```python
from build123d import *

# Parameters (mm, degrees)
BOSS_EXTRUDE1_DEPTH = 20
BOSS_EXTRUDE2_DEPTH = 20
BOSS_EXTRUDE3_DEPTH = 20
SKETCH4_W           = 101.78899744
SKETCH4_H           = 2
SKETCH4_W_2         = 100
SKETCH4_W_3         = 60
SKETCH4_W_4         = 30.536699232
BOSS_EXTRUDE4_DEPTH = 10


with BuildPart() as part:
    # Sketch1 → Boss-Extrude1 (new body)
    with BuildSketch(Plane.XY):
        Polygon((0, 0), (0, 54), (100, 35), (100, 0), align=None)
    extrude(amount=BOSS_EXTRUDE1_DEPTH)

    # Sketch2 → Boss-Extrude2 (add)
    with BuildSketch(Plane.XY.offset(20)):
        Polygon((0, 54), (0, 0), (60, 0), (60, 42.6), align=None)
    extrude(amount=BOSS_EXTRUDE2_DEPTH)

    # Sketch3 → Boss-Extrude3 (add)
    with BuildSketch(Plane.XY.offset(40)):
        Polygon((0, 54), (0, 0), (30, 0), (30, 48.3), align=None)
    extrude(amount=BOSS_EXTRUDE3_DEPTH)

    # Sketch4 → Boss-Extrude4 (add)
    with BuildSketch(Plane(origin=(9.902519062, 52.118521378, 0), x_dir=(0.982424451701422, -0.1866606458232701, 0), z_dir=(0.1866606458232701, 0.982424451701422, 0))):
        with Locations((40.814823846, -1)):
            Rectangle(SKETCH4_W, SKETCH4_H)
        with Locations((39.920325126, -19)):
            Rectangle(SKETCH4_W_2, SKETCH4_H)
        with Locations((19.920325126, -39)):
            Rectangle(SKETCH4_W_3, SKETCH4_H)
        with Locations((5.188674742, -59)):
            Rectangle(SKETCH4_W_4, SKETCH4_H)
    extrude(amount=BOSS_EXTRUDE4_DEPTH)


solid = part.part
```
Build history of the part. All positions in model axes, mm. A direction names the side the tool comes from. Give positions to 0.01 mm unless a question says otherwise; leave off trailing zeros. Loops run counter-clockwise (first coordinate to the right, second up) from the corner with the lowest first, then second, coordinate; pieces in that order, holes last. Notation, with made-up numbers: (0.25, 72) -> (24.25, 72) arc R12 ccw to (24.25, 90) -> close; hole circle Ø1 at (87, 88.5). An arc over 180 degrees is marked (long way). One line per question, with ' | ' between items. Start each with the question number.
1) Cut at A-A (y = 56.5). Give the cut face in (x, z) (3 decimals).
2) Cut at C-C (y = 28). Give the cut face in (x, z).
3) Probe L1, parallel to Z at x = 56, y = 49; L2, parallel to Z at x = 13, y = 53; L3, parallel to X at y = 35, z = 43. List the from-to ranges inside material, lowest first.
4) Two-plate mould, pull along Z, no slides. Class faces 1 (the flat face through (16, 32, 60)), 2 (the flat face through (100, 18, 10)), 3 (the flat face through (16, 56, 58)): released by +Z, released by -Z, zero draft, split by the parting line, or undercut.
5) 3-axis set-ups, long thin cutter, end or side, ignore diameter. For faces 4 (the flat face through (50, 49, 2)), 5 (the flat face through (51.167, 54.457, 0.986)): which of +Z, -Z, +X, -X, +Y, -Y reach the whole face in a straight line?
6) Cut at B-B (x = 45.5). Give the cut face in (y, z) (3 decimals), plus the area to 3 significant figures.
7) Pin check, flat tips, straight feed: pin 1 (12 mm diameter, centred on x = 75, y = 41, fed in from +Z); pin 2 (10 mm diameter, centred on y = 22, z = 45.5, fed in from +X); pin 3 (22 mm diameter, centred on y = 19, z = 34.5, fed in from +X). Stop position of each tip, or through.
8) Cut at D-D (z = 46.5). Give the cut face in (x, y).
Return value:
1) outline: (0.475, 0) -> (40.415, 0) -> (40.415, 2) -> (0.475, 2) -> close; (0.475, 18) -> (40.415, 18) -> (40.415, 20) -> (0.475, 20) -> close; (0.475, 38) -> (40.415, 38) -> (40.415, 40) -> (0.475, 40) -> close; (0.475, 58) -> (31.558, 58) -> (31.558, 60) -> (0.475, 60) -> close
2) outline: (0, 0) -> (100, 0) -> (100, 20) -> (60, 20) -> (60, 40) -> (30, 40) -> (30, 60) -> (0, 60) -> close
3) L1: 0 to 2, 18 to 20, 38 to 40 | L2: 0 to 2, 18 to 20, 38 to 40, 58 to 60 | L3: 0 to 30
4) face 1: released by +Z | face 2: zero draft | face 3: undercut
5) face 4: +X, +Y | face 5: +Z, -Z, +X, +Y
6) outline: (0, 0) -> (55.534, 0) -> (55.534, 2) -> (45.355, 2) -> (45.355, 18) -> (55.534, 18) -> (55.534, 20) -> (45.355, 20) -> (45.355, 38) -> (55.534, 38) -> (55.534, 40) -> (0, 40) -> close | area: 1,880 mm^2
7) pin 1: z = 20 | pin 2: x = 30 | pin 3: x = 60
8) outline: (0, 0) -> (30, 0) -> (30, 48.3) -> (0, 54) -> close
